```python
from build123d import *

# Parameters (mm, degrees)
F1_DEPTH       = 3
F3_D           = 3.3
F3_CSINK_D     = 6.72
F3_CSINK_ANGLE = 90
F4_R           = 8
F5_DEPTH       = 13
F6_SIZE2       = 0.5
F6_SIZE        = 0.5
F7_R           = 5
F8_DEPTH       = 14
F9_R           = 4.5
F10_DEPTH      = 16
F11_SIZE2      = 0.49999
F11_SIZE       = 0.49999
F12_SIZE2      = 2
F12_SIZE       = 2


# Not quite as in the source:
# - a fillet or chamfer is up to 0.001 mm smaller than in the source, because OpenCascade refuses the exact size


with BuildPart() as f1:
    # F0 (on Top) → F1 (new body)
    with BuildSketch(Plane.XY):
        with BuildLine():
            Line((10.8069422132, 8.9), (-10.8069422132, 8.9))
            ThreePointArc((-10.8069422132, 8.9), (-14, 0), (-10.8069422132, -8.9))
            Line((-10.8069422132, -8.9), (10.8069422132, -8.9))
            ThreePointArc((10.8069422132, -8.9), (14, 0), (10.8069422132, 8.9))
        make_face()
    extrude(amount=F1_DEPTH)

    # F3 (through all)
    with Locations(Plane(origin=(0, 0, 0), x_dir=(1, 0, 0), z_dir=(0, 0, -1))):
        with Locations((-10, 0), (10, 0)):
            CounterSinkHole(F3_D / 2, F3_CSINK_D / 2, counter_sink_angle=F3_CSINK_ANGLE)

    # F4 (on face) → F5 (join)
    with BuildSketch(Plane.XY.offset(3)):
        Circle(F4_R)
    extrude(amount=F5_DEPTH)

    # F6
    f6_edges = [f1.edges().sort_by_distance(p)[0] for p in [
        (0, 8.9, 3),
        (14, 0, 3),
        (0, -8.9, 3),
        (-14, 0, 3),
    ]]
    chamfer(f6_edges, length=F6_SIZE, length2=F6_SIZE2)

    # F7 (on face) → F8 (join)
    with BuildSketch(Plane.XY.offset(16)):
        Circle(F7_R)
    extrude(amount=F8_DEPTH)

    # F9 (on face) → F10 (join)
    with BuildSketch(Plane.XY.offset(30)):
        Circle(F9_R)
    extrude(amount=F10_DEPTH)

    # F11 (size 0.5 and 0.5 in the source; OpenCascade refuses exactly that, so slightly less here)
    f11_edges = [f1.edges().sort_by_distance(p)[0] for p in [
        (-5, 0, 30),
        (-8, 0, 16),
        (-5, 0, 16),
        (0, 8.9, 0),
        (14, 0, 0),
        (-14, 0, 0),
        (0, -8.9, 0),
    ]]
    chamfer(f11_edges, length=F11_SIZE, length2=F11_SIZE2)

    # F12
    f12_edges = [f1.edges().sort_by_distance(p)[0] for p in [
        (-4.5, 0, 46),
    ]]
    chamfer(f12_edges, length=F12_SIZE, length2=F12_SIZE2)


solid = f1.part
```
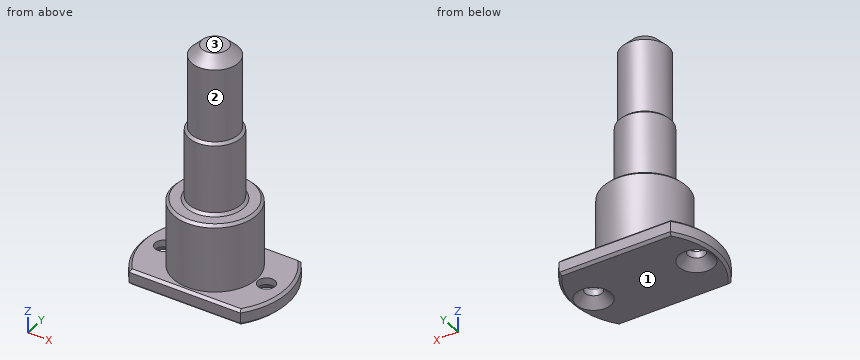
Model file for the job. Use its own axes, mm. Face numbers are marked on the shaded views. Coordinates: 2 decimals unless noted, no trailing zeros. Loops run counter-clockwise (first coordinate to the right, second up) from the corner with the lowest first, then second, coordinate; pieces in that order, holes last. Notation, with made-up numbers: (59.25, 89) - (101.25, 89) arc R22 cw to (101.25, 95) - close; hole circle Ø7 at (33, -33). An arc over 180 degrees is marked (long way). Write item = value, one per line. Start each with the question number.
Item 1: Saw through at A-A, the plane x = -10. List the corners of the cut face in (y, z).
Item 2: Drop flat-ended pins along their axis: pin 1 Ø12 at (x, z) = (-8, 11) entering from -Y; pin 2 Ø3 at (x, y) = (-10, 0) entering from +Z; pin 3 Ø10 at (y, z) = (-4, 33.5) entering from -X; pin 4 Ø6 at (x, z) = (6, 8) entering from -Y. Give the stop position or say it passes through.
Item 3: Saw through at D-D, the plane z = 11. List the corners of the cut face in (x, y), then the cut area to 3 significant figures.
Item 4: Pull direction Z, two halves, no side cores. Call the marked faces 1, 2 and 3: +Z half, -Z half, draft (parallel to the pull), parting line (faces both ways), or undercut.
Item 5: Saw through at C-C, the plane z = 32. List the corners of the cut face in (x, y).
Item 6: Wall check: probe 1 along Y at (x, z) = (10, 2.15); probe 2 along Z at (x, y) = (5.5, 2); probe 3 along Z at (x, y) = (9.5, -3.5). Give the ranges that are in metal, low to high. Write a range as [from, to].
Answers:
q1.outline = (-8.9, 0.5) - (-8.4, 0) - (-3.36, 0) - (-1.65, 1.71) - (-1.65, 3) - (-8.4, 3) - (-8.9, 2.5) - close; (1.65, 1.71) - (3.36, 0) - (8.4, 0) - (8.9, 0.5) - (8.9, 2.5) - (8.4, 3) - (1.65, 3) - close
q2.pin_1 = -7.75
q2.pin_2 = through
q2.pin_3 = -4.9
q2.pin_4 = -7.42
q3.outline = circle Ø16 at (0, 0)
q3.area = 201 mm2
q4.face_1 = -Z half
q4.face_2 = draft
q4.face_3 = +Z half
q5.outline = circle Ø9 at (0, 0)
q6.probe_1 = [-8.9, -1.65], [1.65, 8.9]
q6.probe_2 = [0, 16]
q6.probe_3 = [0, 3]
